The model under review builds one solid part; all positions refer to its coordinate system, in mm. A direction names the side the tool comes from. Give positions to 0.01 mm unless a question says otherwise; leave off trailing zeros. Order: outer loops, then holes, each group sorted by start corner. A loop starts at its lowest first (then second) coordinate and runs counter-clockwise, first axis right, second up. Notation, with made-up numbers: M 25,-28 L 80,-28 A6 cw 80,-20 Z; hole C 1.25,52.5 d3. An arc over 180 degrees is marked long. One line per question, with ' | ' between items. Start each with the question number.
1. We need section B-B on z = 0. Write out the cut boundary in (x, y).
2. Insertion check: P1, Ø8, axis at x = -8, y = 23, coming from the +Z side; P2, Ø4, axis at y = 17.5, z = -7.5, coming from the -X side; P3, Ø6, axis at x = 7.5, y = 12, coming from the -Z side. Each pin has a flat end and moves straight along its axis. Give the tip position at first contact, or say it passes through.
3. Wall thickness on L1, parallel to Z at x = 0, y = 2.7; L2, parallel to Z at x = 0, y = 17.75; L3, parallel to Y at x = -7, z = -2.25: over which ranges is each line inside the solid? List them lowest first.
4. We need section A-A on x = 0. Write out the cut boundary in (y, z), then the cut area to 3 significant figures.
5. We need section C-C on y = 5. Write out the cut boundary in (x, z).
6. For faces 5 (the face through (12, 0, 2)), 6 (the face through (11.446, 0.986, -3.604)), 7 (the face through (7, 3, -10)), list the 3-axis set-ups (+Z, -Z, +X, -X, +Y, -Y) from which the entire face can be reached by the end or side of a thin tool; tool diameter is ignored.
7. The part is to be moulded in two halves that separate along Z. For faces 1 (the face through (11.923, 2.493, -3.755)), 2 (the face through (0, 28.8, 0)), 3 (the face through (-2.93, 13.59, 13.18)), 4 (the face through (0, 25.8, 0)), say which applies: +Z half, -Z half, draft (parallel to the pull), parting line (faces both ways), or undercut.
```python
from build123d import *

# Parameters (mm, degrees)
CONG_1_R = 2


with BuildPart() as part:
    # Esquisse1 → Révolution1 (revolve)
    with BuildSketch(Plane.XY, mode=Mode.PRIVATE) as r_volution1_sk:
        Polygon((-13.5, 0), (-13.5, 28.8), (0, 28.8), (0, 25.8), (-12, 25.8), (-12, 3), (-12.5, 3), (-12.5, 2), (-12, 2), (-12, 0), align=None)
    revolve(r_volution1_sk.sketch.rotate(Axis((0, 0, 0), (0, 1, 0)), 180), axis=Axis((0, 0, 0), (0, 1, 0)))

    # Congé1
    cong_1_edges = [part.edges().sort_by_distance(p)[0] for p in [
        (-13.5, 28.8, 0),
    ]]
    fillet(cong_1_edges, radius=CONG_1_R)


solid = part.part
```
Entries:
1) outline: M -13.5,0 L -12,0 L -12,2 L -12.5,2 L -12.5,3 L -12,3 L -12,25.8 L 12,25.8 L 12,3 L 12.5,3 L 12.5,2 L 12,2 L 12,0 L 13.5,0 L 13.5,26.8 A2 ccw 11.5,28.8 L -11.5,28.8 A2 ccw -13.5,26.8 Z
2) P1: stops at z = 12.89 | P2: stops at x = -12.33 | P3: stops at z = -12.73
3) L1: z = -13.5 to -12.5, 12.5 to 13.5 | L2: z = -13.5 to -12, 12 to 13.5 | L3: y = 25.8 to 28.8
4) outline: M 0,-13.5 L 26.8,-13.5 A2 ccw 28.8,-11.5 L 28.8,11.5 A2 ccw 26.8,13.5 L 0,13.5 L 0,12 L 2,12 L 2,12.5 L 3,12.5 L 3,12 L 25.8,12 L 25.8,-12 L 3,-12 L 3,-12.5 L 2,-12.5 L 2,-12 L 0,-12 Z | area: 156 mm^2
5) outline: C 0,0 d27; hole C 0,0 d24
6) face 5: +Z, -Z, +X, -X, -Y | face 6: -Y | face 7: none
7) face 1: undercut | face 2: draft | face 3: parting line | face 4: undercut
